from build123d import *

# Parameters (mm, degrees)
BOSS_EXTRUDE1_DEPTH                               = 20
CBORE_FOR_M4_SHCS1_D                              = 4.5
CBORE_FOR_M4_SHCS1_CBORE_D                        = 8
CBORE_FOR_M4_SHCS1_CBORE_DEPTH                    = 4
CSK_FOR_8_FLAT_HEAD_SOCKET_CAP_SCREW1_D           = 4.4958
CSK_FOR_8_FLAT_HEAD_SOCKET_CAP_SCREW1_CSINK_D     = 10.16
CSK_FOR_8_FLAT_HEAD_SOCKET_CAP_SCREW1_CSINK_ANGLE = 82
BOSS_EXTRUDE2_DEPTH                               = 3
BOSS_EXTRUDE3_START                               = -20
BOSS_EXTRUDE3_DEPTH                               = 3


with BuildPart() as part:
    # Sketch1 → Boss-Extrude1 (new body)
    with BuildSketch(Plane(origin=(0, 0, 0), x_dir=(1, 0, 0), z_dir=(0, 1, 0))):
        Polygon((0, 0), (0, 11), (7, 11), (7, -7), (-18, -7), (-18, 0), align=None)
    extrude(amount=BOSS_EXTRUDE1_DEPTH)

    # CBORE for M4 SHCS1 (through all)
    with Locations(Plane.ZY):
        with Locations((-5.5, 10)):
            CounterBoreHole(CBORE_FOR_M4_SHCS1_D / 2, CBORE_FOR_M4_SHCS1_CBORE_D / 2, CBORE_FOR_M4_SHCS1_CBORE_DEPTH)

    # CSK for #8 Flat Head Socket Cap Screw1 (through all)
    with Locations(Plane(origin=(0, 0, 0), x_dir=(-1, 0, 0), z_dir=(0, 0, -1))):
        with Locations((9, 10)):
            CounterSinkHole(CSK_FOR_8_FLAT_HEAD_SOCKET_CAP_SCREW1_D / 2, CSK_FOR_8_FLAT_HEAD_SOCKET_CAP_SCREW1_CSINK_D / 2, counter_sink_angle=CSK_FOR_8_FLAT_HEAD_SOCKET_CAP_SCREW1_CSINK_ANGLE)

    # Sketch6 → Boss-Extrude2 (add)
    with BuildSketch(Plane.XZ):
        Polygon((-18, 7), (7, 7), (7, -11), (0, -11), (-18, 0), align=None)
    extrude(amount=BOSS_EXTRUDE2_DEPTH)

    # Sketch6<2> → Boss-Extrude3 (add)
    with BuildSketch(Plane.XZ.offset(BOSS_EXTRUDE3_START)):
        Polygon((-18, 7), (7, 7), (7, -11), (0, -11), (-18, 0), align=None)
    extrude(amount=-BOSS_EXTRUDE3_DEPTH)


solid = part.part
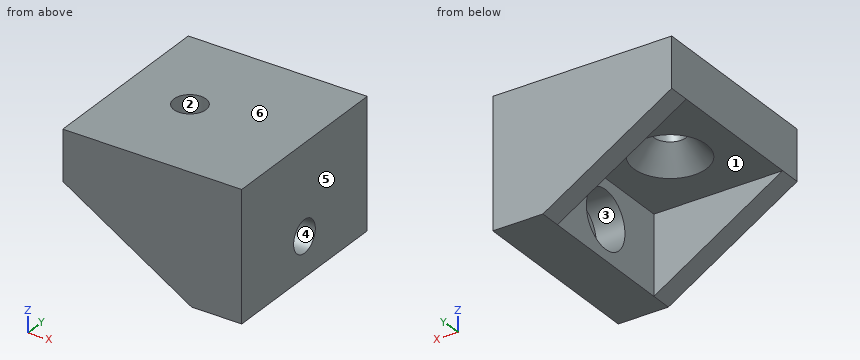
For this review, take the finished solid that the model builds, in its own axes (mm). Face numbers are marked on the shaded views. A direction names the side the tool comes from. Round coordinates to 2 decimals unless told otherwise and drop trailing zeros. Order: outer loops, then holes, each group sorted by start corner. A loop starts at its lowest first (then second) coordinate and runs counter-clockwise, first axis right, second up. Notation, with made-up numbers: (23, 10.5) -> (55, 10.5) arc R19 ccw to (55, 33.5) -> close; hole circle Ø10 at (56, 12.25). An arc over 180 degrees is marked (long way). Put each result on its own line as item: value.
Q1. Add section A-A on y = 10. Write out the cut boundary in (x, z), plus the area to 3 significant figures.
Check result:
outline: (-18, 0) -> (-14.08, 0) -> (-11.25, 3.26) -> (-11.25, 7) -> (-18, 7) -> close; (-6.75, 3.26) -> (-3.92, 0) -> (0, 0) -> (0, -1.5) -> (4, -1.5) -> (4, -3.25) -> (7, -3.25) -> (7, 7) -> (-6.75, 7) -> close; (0, -11) -> (7, -11) -> (7, -7.75) -> (4, -7.75) -> (4, -9.5) -> (0, -9.5) -> close
area: 166 mm2
Q2. For probe 1 along Y at (x, z) = (-8.5, -0.25); probe 2 along Y at (x, z) = (-9, 5.3); probe 3 along X at (y, z) = (10, 6.25), list the stretches that pass through material, from the lowest coordinate up. Write a range as [from, to].
Check result:
probe 1: [-3, 0], [20, 23]
probe 2: [-3, 7.75], [12.25, 23]
probe 3: [-18, -11.25], [-6.75, 7]
Q3. Machinability: for the marked faces 1, 2 and 3, which of the approach directions +Z, -Z, +X, -X, +Y, -Y give a long, thin tool a straight path to every point of the face, cutting with its end or side? Answer none if there is none.
Check result:
face 1: -Z, -X
face 2: +Z, -Z
face 3: -X
Q4. Add section C-C on z = -5.5. Write out the cut boundary in (x, y), plus the area to 4 significant figures.
Check result:
outline: (-9, -3) -> (7, -3) -> (7, 7.75) -> (4, 7.75) -> (4, 6) -> (0, 6) -> (0, 0) -> (-9, 0) -> close; (-9, 20) -> (0, 20) -> (0, 14) -> (4, 14) -> (4, 12.25) -> (7, 12.25) -> (7, 23) -> (-9, 23) -> close
area: 190.5 mm2
Q5. Mouldability with a two-part tool opening along Z and no side actions: class the marked faces 4, 5 and 6 as pulls with the +Z half, pulls with the -Z half, needs draft (parallel to the pull), parting line crosses it, or undercut.
Check result:
face 4: undercut
face 5: needs draft
face 6: pulls with the +Z half
Q6. Insertion check: pin 1 Ø9 at (x, y) = (-12, 8) entering from -Z; pin 2 Ø7 at (y, z) = (10, -5.5) entering from -X; pin 3 Ø7 at (x, y) = (-9, 10) entering from -Z. Each pin has a flat end and moves straight along its axis. Give the tip position at first contact, or say it passes through.
Check result:
pin 1: z = 0
pin 2: x = 4
pin 3: z = 1.82
Q7. Add section D-D on z = 6.25. Write out the cut boundary in (x, y).
Check result:
outline: (-18, -3) -> (7, -3) -> (7, 23) -> (-18, 23) -> close; hole circle Ø4.5 at (-9, 10)
Q8. Add section B-B on x = -9. Write out the cut boundary in (y, z).
Check result:
outline: (-3, -5.5) -> (0, -5.5) -> (0, 0) -> (4.92, 0) -> (7.75, 3.26) -> (7.75, 7) -> (-3, 7) -> close; (12.25, 3.26) -> (15.08, 0) -> (20, 0) -> (20, -5.5) -> (23, -5.5) -> (23, 7) -> (12.25, 7) -> close
